Verification items for the finished model (mm, model axes). A direction names the side the tool comes from. Round coordinates to 2 decimals unless told otherwise and drop trailing zeros. Loops run counter-clockwise (first coordinate to the right, second up) from the corner with the lowest first, then second, coordinate; pieces in that order, holes last. Notation, with made-up numbers: (-15, -36) -> (43, -36) arc R10 ccw to (43, -28) -> close; hole circle Ø2 at (-11, 24). An arc over 180 degrees is marked (long way). Write item = value, one per line.
```python
from build123d import *

# Parameters (mm, degrees)
BOSS_EXTRUDE1_DEPTH = 5
CUT_EXTRUDE1_DEPTH  = 10
SKETCH3_W           = 5
SKETCH3_H           = 5
SKETCH3_W_2         = 15
BOSS_EXTRUDE2_DEPTH = 5
SKETCH5_W           = 10
SKETCH5_H           = 30
BOSS_EXTRUDE3_DEPTH = 2.5
SKETCH6_W           = 5.9
SKETCH6_H           = 4.637740471
SKETCH6_H_2         = 12.862259529
SKETCH6_W_2         = 5
SKETCH6_H_3         = 2
SKETCH6_W_3         = 2
SKETCH6_H_4         = 3.737740471
SKETCH6_H_5         = 1.262259529
BOSS_EXTRUDE6_DEPTH = 5
SKETCH7_W           = 0.9
SKETCH7_H           = 22.5
BOSS_EXTRUDE7_DEPTH = 5
SKETCH8_W           = 11.8
SKETCH8_H           = 22.5
CUT_EXTRUDE2_DEPTH  = 5
SKETCH9_W           = 15.8
SKETCH9_H           = 26.5
SKETCH9_W_2         = 11.8
SKETCH9_H_2         = 22.5
BOSS_EXTRUDE8_DEPTH = 6


with BuildPart() as part:
    # Sketch1 → Boss-Extrude1 (new body)
    with BuildSketch(Plane.XY):
        Polygon((-37.5, 25), (-112.5, 125), (-62.5, 25), align=None)
        with BuildLine():
            Line((-37.5, 25), (-62.5, 25))
            Line((-62.5, 25), (-62.5, -25))
            Line((-62.5, -25), (62.5, -25))
            Line((62.5, -25), (62.5, 25))
            Line((62.5, 25), (37.5, 25))
            ThreePointArc((37.5, 25), (0, -12.5), (-37.5, 25))
        make_face()
        Polygon((112.5, 125), (37.5, 25), (62.5, 25), align=None)
    extrude(amount=BOSS_EXTRUDE1_DEPTH)

    # Sketch2 → Cut-Extrude1 (cut)
    with BuildSketch(Plane.XY.offset(5)):
        Polygon((42.5, -15), (-42.5, -15), (-42.5, 25), (-57.5, 25), (-57.5, -20), (57.5, -20), (57.5, 25), (42.5, 25), align=None)
        Polygon((-57.5, 25), (-42.5, 25), (-99.706643081, 105), align=None)
        Polygon((101.413859584, 108.353754457), (42.5, 25), (57.5, 25), align=None)
    extrude(amount=-CUT_EXTRUDE1_DEPTH, mode=Mode.SUBTRACT)

    # Sketch3 → Boss-Extrude2 (add)
    with BuildSketch(Plane.XY.offset(5)):
        with Locations((-28.877625422, -17.5)):
            Rectangle(SKETCH3_W, SKETCH3_H)
        with Locations((22.225490127, -17.5)):
            Rectangle(SKETCH3_W, SKETCH3_H)
        with Locations((50, 8.762259529)):
            Rectangle(SKETCH3_W_2, SKETCH3_H)
        with Locations((-50, 8.762259529)):
            Rectangle(SKETCH3_W_2, SKETCH3_H)
        Polygon((-70.654305037, 49.93314621), (-63.796030498, 54.781199316), (-66.704368337, 58.848332338), (-72.987424539, 54.355425418), align=None)
        Polygon((65.786619226, 57.946867762), (62.925217298, 53.89843849), (70.065851227, 48.851487608), (72.396389437, 53.275127699), align=None)
    extrude(amount=-BOSS_EXTRUDE2_DEPTH)

    # Sketch5 → Boss-Extrude3 (add)
    with BuildSketch(Plane(origin=(0, 0, 0), x_dir=(-1, 0, 0), z_dir=(0, 0, -1))):
        with Locations((-32.5, -40)):
            Rectangle(SKETCH5_W, SKETCH5_H)
    extrude(amount=-BOSS_EXTRUDE3_DEPTH)

    # Sketch6 → Boss-Extrude6 (add)
    with BuildSketch(Plane.XY.offset(5)):
        with Locations((54.55, 13.581129765)):
            Rectangle(SKETCH6_W, SKETCH6_H)
        Polygon((51.6, 11.262259529), (51.6, 10), (57.5, 10), (62.5, 10), (62.5, 15.9), (57.5, 15.9), (57.5, 11.262259529), align=None)
        Polygon((57.5, 10), (51.6, 10), (51.6, 6.262259529), (57.5, 6.262259529), (57.5, -6.6), (62.5, -6.6), (62.5, 10), align=None)
        with Locations((54.55, -0.168870236)):
            Rectangle(SKETCH6_W, SKETCH6_H_2)
        Polygon((63.4, 15.9), (63.4, 10), (63.4, -6.6), (62.5, -6.6), (62.5, -8.6), (65.4, -8.6), (65.4, 17.9), (62.5, 17.9), (62.5, 15.9), align=None)
        with Locations((60, 16.9)):
            Rectangle(SKETCH6_W_2, SKETCH6_H_3)
        Polygon((49.6, 11.262259529), (51.6, 11.262259529), (51.6, 15.9), (57.5, 15.9), (57.5, 17.9), (49.6, 17.9), align=None)
        Polygon((51.6, -6.6), (51.6, 6.262259529), (49.6, 6.262259529), (49.6, -8.6), (57.5, -8.6), (57.5, -6.6), align=None)
        with Locations((60, -7.6)):
            Rectangle(SKETCH6_W_2, SKETCH6_H_3)
        with Locations((50.6, 8.131129765)):
            Rectangle(SKETCH6_W_3, SKETCH6_H_4)
        with Locations((50.6, 10.631129765)):
            Rectangle(SKETCH6_W_3, SKETCH6_H_5)
    extrude(amount=-BOSS_EXTRUDE6_DEPTH)

    # Sketch7 → Boss-Extrude7 (add)
    with BuildSketch(Plane.XY.offset(5)):
        with Locations((62.95, 4.65)):
            Rectangle(SKETCH7_W, SKETCH7_H)
    extrude(amount=-BOSS_EXTRUDE7_DEPTH)

    # Sketch8 → Cut-Extrude2 (cut)
    with BuildSketch(Plane.XY.offset(5)):
        with Locations((57.5, 4.65)):
            Rectangle(SKETCH8_W, SKETCH8_H)
    extrude(amount=-CUT_EXTRUDE2_DEPTH, mode=Mode.SUBTRACT)

    # Sketch9 → Boss-Extrude8 (add)
    with BuildSketch(Plane.XY.offset(5)):
        with Locations((57.5, 4.65)):
            Rectangle(SKETCH9_W, SKETCH9_H)
        with Locations((57.5, 4.65)):
            Rectangle(SKETCH9_W_2, SKETCH9_H_2, mode=Mode.SUBTRACT)
    extrude(amount=BOSS_EXTRUDE8_DEPTH)


solid = part.part
```
(1) Set-up check for faces 1 (the face through (-42.5, 18, 3)), 2 (the face through (62.5, 21, 2)), 3 (the face through (49.6, 4, 5)): record each of +Z, -Z, +X, -X, +Y, -Y from which the full face is reachable in a straight line by a thin tool's end or side.
Filled sheet:
face_1 = +Z, -Z
face_2 = +Z, -Z, +X
face_3 = +Z
(2) Sectioned sample at A-A, the plane x = 0. Record the cut outline in (y, z), and give its area (3 significant figures).
Filled sheet:
outline = (-25, 0) -> (-20, 0) -> (-20, 5) -> (-25, 5) -> close; (-15, 0) -> (-12.5, 0) -> (-12.5, 5) -> (-15, 5) -> close
area = 37.5 mm2
(3) Go/stop test with flat-tipped pins: pin 1 Ø3 at (x, z) = (50, 7) entering from -Y; pin 2 Ø2.5 at (x, z) = (-7, 3.5) entering from +Y; pin 3 Ø4 at (y, z) = (-18.5, 3) entering from -X. Record where each tip stops, or that it passes through.
Filled sheet:
pin_1 = -8.6
pin_2 = -11.58
pin_3 = -62.5
(4) Draft check along Y on faces 4 (the face through (-88, 76, 2)), 5 (the face through (34, -15, 3)), 6 (the face through (50, 5, 11)). Enter one of: released by +Y, released by -Y, zero draft, split by the parting line, or undercut.
Filled sheet:
face_4 = released by -Y
face_5 = undercut
face_6 = zero draft
(5) Sectioned sample at C-C, the plane y = -44. Record the cut outline in (x, z).
Filled sheet:
outline = (27.5, 0) -> (37.5, 0) -> (37.5, 2.5) -> (27.5, 2.5) -> close
(6) Sectioned sample at B-B, the plane z = 6.75. Record the cut outline in (x, y), and give its area (3 significant figures).
Filled sheet:
outline = (49.6, -8.6) -> (65.4, -8.6) -> (65.4, 17.9) -> (49.6, 17.9) -> close; hole (51.6, -6.6) -> (63.4, -6.6) -> (63.4, 15.9) -> (51.6, 15.9) -> close
area = 153 mm2
(7) Material ranges on probe 1 along X at (y, z) = (26, 1.5); probe 2 along X at (y, z) = (7, 9); probe 3 along X at (y, z) = (-36.5, 0.75), recorded low to high. Write a range as from..to.
Filled sheet:
probe_1 = -63..-58.03, -43.22..-38.25, 38.25..43.21, 58.03..63
probe_2 = 49.6..51.6, 63.4..65.4
probe_3 = 27.5..37.5
